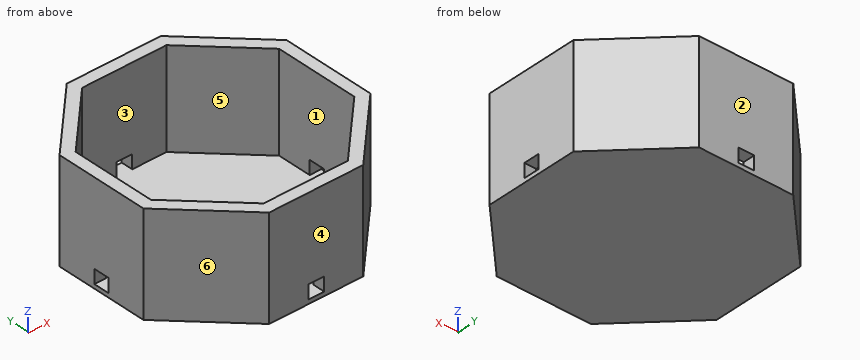
from build123d import *

# Parameters (mm, degrees)
BOSS_EXTRUDE1_DEPTH   = 3
BOSS_EXTRUDE2_DEPTH   = 70
CUT_EXTRUDE1_DEPTH    = 170
SKETCH4_W             = 11.5
SKETCH4_H             = 10
CUT_EXTRUDE2_DEPTH    = 170
BODY_MOVE_COPY2_ANGLE = 90


with BuildPart() as part:
    # Sketch1 → Boss-Extrude1 (new body)
    with BuildSketch(Plane(origin=(0, 0, 0), x_dir=(1, 0, 0), z_dir=(0, 1, 0))):
        Polygon((0, -82), (0, 0), (-82, 0), (-82, -33.965), (-33.964997557, -82), align=None)
        Polygon((82, 0), (0, 0), (0, -82), (33.965002443, -82), (82, -33.965), align=None)
        Polygon((-82, 0), (0, 0), (82, 0), (82, 33.965), (33.965002443, 82), (-33.964997557, 82), (-82, 33.965), align=None)
    extrude(amount=BOSS_EXTRUDE1_DEPTH)

    # Sketch2 → Boss-Extrude2 (add)
    with BuildSketch(Plane(origin=(0, 3, 0), x_dir=(1, 0, 0), z_dir=(0, 1, 0))):
        Polygon((33.965002443, -82), (82, -33.965), (82, 33.965), (33.965002443, 82), (-33.964997557, 82), (-82, 33.965), (-82, -33.965), (-33.964997557, -82), align=None)
        Polygon((-30.44418472, 73.5), (30.44418472, 73.5), (73.5, 30.44418472), (73.5, -30.44418472), (30.44418472, -73.5), (-30.44418472, -73.5), (-73.5, -30.44418472), (-73.5, 30.44418472), align=None, mode=Mode.SUBTRACT)
    extrude(amount=BOSS_EXTRUDE2_DEPTH)

    # Sketch3 → Cut-Extrude1 (cut)
    with BuildSketch(Plane(origin=(82, 0, 0), x_dir=(0, 0, -1), z_dir=(1, 0, 0))):
        Polygon((-5.75, 13), (-5.75, 3), (0, 3), (5.75, 3), (5.75, 13), align=None)
    extrude(amount=-CUT_EXTRUDE1_DEPTH, mode=Mode.SUBTRACT)

    # Sketch4 → Cut-Extrude2 (cut)
    with BuildSketch(Plane(origin=(0, 0, -82), x_dir=(-1, 0, 0), z_dir=(0, 0, -1))):
        with Locations((0, 8)):
            Rectangle(SKETCH4_W, SKETCH4_H)
    extrude(amount=-CUT_EXTRUDE2_DEPTH, mode=Mode.SUBTRACT)


with BuildPart() as part_1:
    # Body-Move/Copy2: moved
    add(part.part.rotate(Axis((0, 36.5, 0), (1, 0, 0)), BODY_MOVE_COPY2_ANGLE))


solid = part_1.part
Build history of the part. All positions in model axes, mm. Face numbers are marked on the shaded views. A direction names the side the tool comes from. Coordinates: 2 decimals unless noted, no trailing zeros. Write each loop counter-clockwise with the first axis right and the second up, starting at its lowest first coordinate (ties: lowest second). Pieces come first, ordered by that corner, then holes.
(1) 3-axis set-ups, long thin cutter, end or side, ignore diameter. For the marked faces 1 and 2: which of +Z, -Z, +X, -X, +Y, -Y reach the whole face in a straight line?
(2) Cut at C-C on x = 9. List the corners of the cut face in (y, z), and give its area (3 significant figures).
(3) Mould opens along X. For the marked faces 3, 4, 5 and 6 say: pulls with the +X half, pulls with the -X half, needs draft (parallel to the pull), parting line crosses it, or undercut.
(4) Cut at B-B on y = 21. List the corners of the cut face in (x, z), and give its area (3 significant figures).
(5) Cut at A-A on z = -20. List the corners of the cut face in (x, y) (3 decimals).
(6) Drill centre lines: line 1 (X direction, y = 15, z = 13); line 2 (Y direction, x = -7, z = -23.5); line 3 (Z direction, x = 40.5, y = 86). Where is each one in solid material? Low to high.
(7) Pin check, flat tips, straight feed: pin 1 Ø7 at (x, z) = (77.5, -28.5) entering from -Y (3 decimals); pin 2 Ø12 at (x, y) = (-51, 56) entering from +Z; pin 3 Ø6 at (x, z) = (-42, -26) entering from +Y (3 decimals). Stop position of each tip, or through.
Working result:
1. face 1: +Z
1. face 2: +Z, -Z, +X, -X, +Y
2. outline: (-45.5, -36.5) - (118.5, -36.5) - (118.5, 36.5) - (110, 36.5) - (110, -33.5) - (-37, -33.5) - (-37, 36.5) - (-45.5, 36.5) - close
2. area: 1,680 mm2
3. face 3: undercut
3. face 4: needs draft
3. face 5: undercut
3. face 6: pulls with the -X half
4. outline: (-82, -36.5) - (82, -36.5) - (82, 36.5) - (73.5, 36.5) - (73.5, -33.5) - (-73.5, -33.5) - (-73.5, 36.5) - (-82, 36.5) - close
4. area: 1,680 mm2
5. outline: (-82, 2.535) - (-33.965, -45.5) - (33.965, -45.5) - (82, 2.535) - (82, 70.465) - (33.965, 118.5) - (-33.965, 118.5) - (-82, 70.465) - close; hole (-73.5, 6.056) - (-30.444, -37) - (30.444, -37) - (73.5, 6.056) - (73.5, 66.944) - (30.444, 110) - (-30.444, 110) - (-73.5, 66.944) - close
6. line 1: x = -82 to -73.5, 73.5 to 82
6. line 2: y = -45.5 to -37, 110 to 118.5
6. line 3: z = -36.5 to -33.5
7. pin 1: stops at y = -5.465
7. pin 2: stops at z = -33.5
7. pin 3: stops at y = 113.465
